Source: three-view drawing plus pictorial views. Frame: mm from the lowest corner of the part. Give positions to 0.01 mm unless a question says otherwise; leave off trailing zeros. Loops run counter-clockwise (first coordinate to the right, second up) from the corner with the lowest first, then second, coordinate; pieces in that order, holes last. Notation, with made-up numbers: M -13.75,-12 L 16.25,-12 A21 cw 16.25,-6 Z; hole C 28,-8.5 d11. An arc over 180 degrees is marked long. Write item = value, one per line.
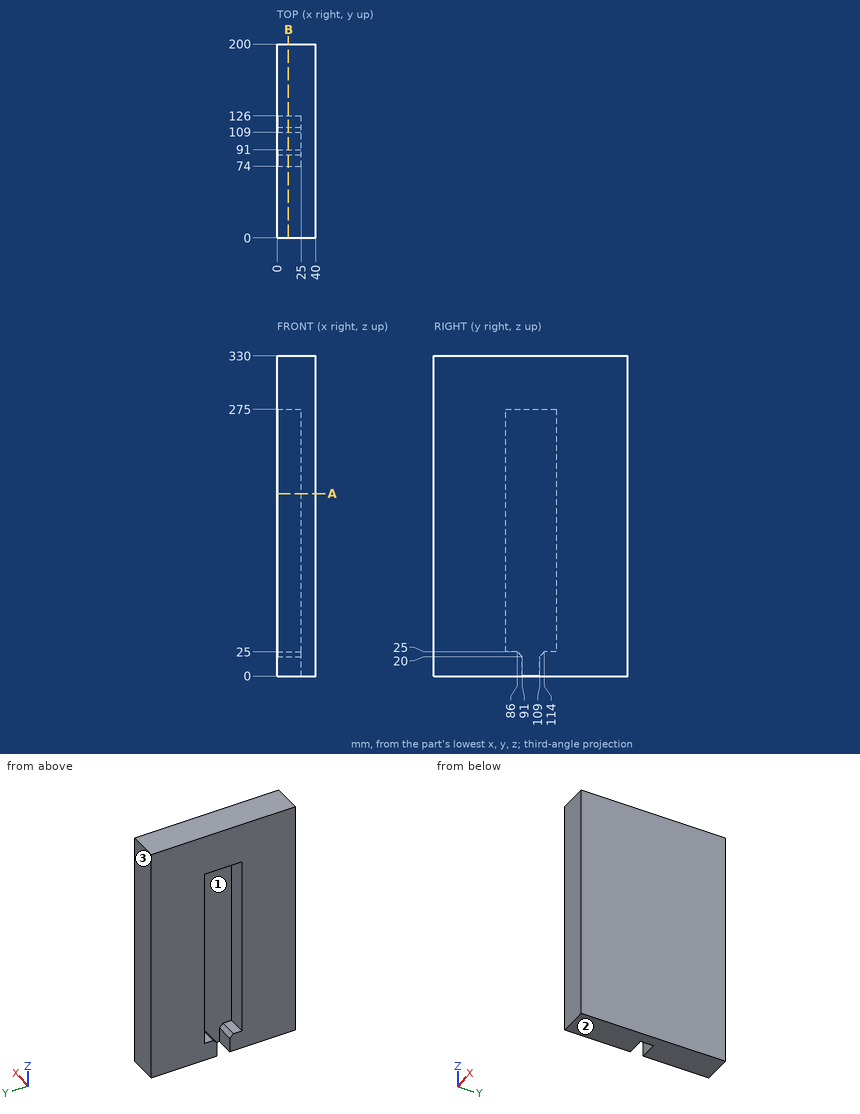
1. Material intervals for probe 1 along Y at (x, z) = (23.5, 75); probe 2 along Z at (x, y) = (23.5, 84); probe 3 along X at (y, z) = (90, 92), sorted ascending. Write a range as from..to.
Derived:
probe_1 = 0..74, 126..200
probe_2 = 0..25, 275..330
probe_3 = 25..40
2. Pull-direction query (Y, two-part tool) for the marked faces 1, 2 and 3; classes: +Y half, -Y half, draft (parallel to the pull), parting line (faces both ways), or undercut.
Derived:
face_1 = undercut
face_2 = draft
face_3 = +Y half
3. Cut plane B-B, the plane x = 11.5. Return the cut outline in (y, z), then the cut area to 3 significant figures.
Derived:
outline = M 0,0 L 91,0 L 91,20 L 86,25 L 74,25 L 74,275 L 126,275 L 126,25 L 114,25 L 109,20 L 109,0 L 200,0 L 200,330 L 0,330 Z
area = 52,500 mm²
4. First-contact query: pin 1 Ø7.5 at (x, y) = (13.5, 101.5) entering from -Z. Flat tip, straight axial feed; report the tip coordinate or a pass-through.
Derived:
pin_1 = 275
5. Cut plane A-A, the plane z = 188. Return the cut outline in (x, y).
Derived:
outline = M 0,0 L 40,0 L 40,200 L 0,200 L 0,126 L 25,126 L 25,74 L 0,74 Z
